Check sheet for the modelled part. Datum: model origin and axes. Units: mm. A direction names the side the tool comes from. Coordinates: 2 decimals unless noted, no trailing zeros. Write each loop counter-clockwise with the first axis right and the second up, starting at its lowest first coordinate (ties: lowest second). Pieces come first, ordered by that corner, then holes. Notation, with made-up numbers: (-10, -24.5) - (3, -24.5) arc R25 cw to (3, 1.5) - close; hole circle Ø7 at (16.25, 69.5). An arc over 180 degrees is marked (long way). Use one line per item in the form item = value. Start each with the question number.
1. Cross-section at C-C on z = 5. Record the boundary of the cut face in (x, y).
2. Cross-section at B-B on z = 11.25. Record the boundary of the cut face in (x, y), then the cut area to 3 significant figures.
3. Cross-section at A-A on x = 0. Record the boundary of the cut face in (y, z), then the cut area to 3 significant figures.
4. Go/stop test with flat-tipped pins: pin 1 Ø1 at (x, y) = (-9.5, 9.5) entering from -Z; pin 2 Ø7.5 at (x, z) = (-13, 10) entering from +Y; pin 3 Ø3 at (y, z) = (13.5, 8.5) entering from -X. Record where each tip stops, or that it passes through.
5. Tool access check on faces 1 (the face through (9, 13, 10)), 2 (the face through (-9, 13, 10)), 3 (the face through (16, 5, 10)). Record the directions out of +Z, -Z, +X, -X, +Y, -Y that give a thin tool (end or side, any length) a straight path to the whole face; none if there is none.
6. Scan lines: line 1 along Z through (x, y) = (0, 13.75); line 2 along Y through (x, z) = (12.5, 6.5); line 3 along X through (y, z) = (14.75, 1.5). Record each from-to range of solid material in increasing order.
7. Cross-section at D-D on y = 6. Record the boundary of the cut face in (x, z).
8. Draft check along Z on faces 4 (the face through (0, 6, 21.082)), 5 (the face through (3.149, 8.061, 12.956)), 6 (the face through (0, 6, 0)). Enter one of: +Z half, -Z half, draft (parallel to the pull), parting line (faces both ways), or undercut.
```python
from build123d import *

# Parameters (mm, degrees)
BOSS_EXTRUDE1_DEPTH     = 21.082
F_3_8_16_TAPPED_HOLE1_D = 7.9375


with BuildPart() as part:
    # Sketch1 → Boss-Extrude1 (new body)
    with BuildSketch(Plane.XY):
        Polygon((-16, 0), (16, 0), (16, 10), (9, 10), (9, 16.35), (-9, 16.35), (-9, 10), (-16, 10), align=None)
    extrude(amount=BOSS_EXTRUDE1_DEPTH)

    # 3/8-16 Tapped Hole1 (through all)
    with Locations(Plane(origin=(0, 16.35, 0), x_dir=(1, 0, 0), z_dir=(0, 1, 0))):
        with Locations((0, -10.541)):
            Hole(F_3_8_16_TAPPED_HOLE1_D / 2)


solid = part.part
```
Final values:
q1.outline = (-16, 0) - (16, 0) - (16, 10) - (9, 10) - (9, 16.35) - (-9, 16.35) - (-9, 10) - (-16, 10) - close
q2.outline = (-16, 0) - (-3.9, 0) - (-3.9, 16.35) - (-9, 16.35) - (-9, 10) - (-16, 10) - close; (3.9, 0) - (16, 0) - (16, 10) - (9, 10) - (9, 16.35) - (3.9, 16.35) - close
q2.area = 307 mm²
q3.outline = (0, 0) - (16.35, 0) - (16.35, 6.57) - (0, 6.57) - close; (0, 14.51) - (16.35, 14.51) - (16.35, 21.08) - (0, 21.08) - close
q3.area = 215 mm²
q4.pin_1 = 0
q4.pin_2 = 10
q4.pin_3 = -9
q5.face_1 = +Z, -Z, +X, +Y
q5.face_2 = +Z, -Z, -X, +Y
q5.face_3 = +Z, -Z, +X, +Y, -Y
q6.line_1 = 0 to 6.57, 14.51 to 21.08
q6.line_2 = 0 to 10
q6.line_3 = -9 to 9
q7.outline = (-16, 0) - (16, 0) - (16, 21.08) - (-16, 21.08) - close; hole circle Ø7.94 at (0, 10.54)
q8.face_4 = +Z half
q8.face_5 = undercut
q8.face_6 = -Z half
